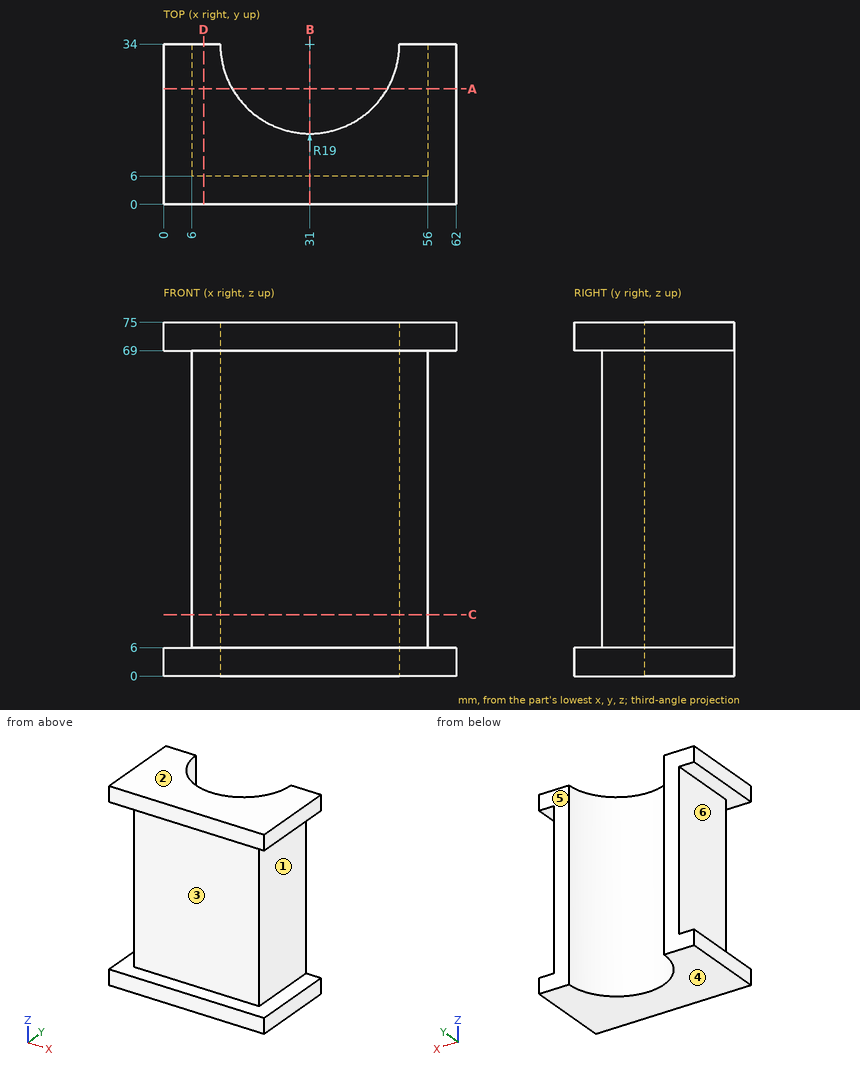
Design review of the part shown in the three views and the two pictorial views. Dimensions are in mm from the part's minimum x, y and z. A direction names the side the tool comes from. Round coordinates to 2 decimals unless told otherwise and drop trailing zeros. Order: outer loops, then holes, each group sorted by start corner. A loop starts at its lowest first (then second) coordinate and runs counter-clockwise, first axis right, second up. Notation, with made-up numbers: (47, 44.5) - (89, 44.5) arc R32 cw to (89, 79.5) - close; hole circle Ø4 at (54.25, 22.25). An arc over 180 degrees is marked (long way). Answer in a Markdown table with one row per item.
(1) Take a section at A-A on y = 24.5. Write out the cut boundary in (x, z), plus the area to 3 significant figures.
Result set:
| item | result |
|---|---|
| outline | (0, 0) - (14.55, 0) - (14.55, 75) - (0, 75) - (0, 69) - (6, 69) - (6, 6) - (0, 6) - close; (47.45, 0) - (62, 0) - (62, 6) - (56, 6) - (56, 69) - (62, 69) - (62, 75) - (47.45, 75) - close |
| area | 1,430 mm2 |
(2) For line 1 (Z direction, x = 44.5, y = 5.5); line 2 (X direction, y = 31.5, z = 12); line 3 (X direction, y = 9, z = 61.5), list the stretches that pass through material, from the lowest coordinate up. Write a range as from..to.
Result set:
| item | result |
|---|---|
| line 1 | z = 0..6, 69..75 |
| line 2 | x = 6..12.17, 49.83..56 |
| line 3 | x = 6..56 |
(3) Take a section at C-C on z = 13. Write out the cut boundary in (x, y), plus the area to 3 significant figures.
Result set:
| item | result |
|---|---|
| outline | (6, 6) - (56, 6) - (56, 34) - (50, 34) arc R19 cw to (12, 34) - (6, 34) - close |
| area | 833 mm2 |
(4) Mouldability with a two-part tool opening along Z and no side actions: class the marked faces 4, 5 and 6 as released by +Z, released by -Z, zero draft, split by the parting line, or undercut.
Result set:
| item | result |
|---|---|
| face 4 | released by -Z |
| face 5 | zero draft |
| face 6 | undercut |
(5) Clearance check with flat-ended pins moving along their axes: P1, Ø8.5, axis at y = 22, z = 26, coming from the +X side; P2, Ø2, axis at y = 16.5, z = 8, coming from the -X side; P3, Ø6, axis at x = 17.5, z = 8.5, coming from the +Y side. State where each tip first meets the part, or that it passes through.
Result set:
| item | result |
|---|---|
| P1 | stops at x = 56 |
| P2 | stops at x = 6 |
| P3 | stops at y = 24.58 |
(6) Take a section at B-B on x = 31. Write out the cut boundary in (y, z), plus the area to 3 significant figures.
Result set:
| item | result |
|---|---|
| outline | (0, 0) - (15, 0) - (15, 75) - (0, 75) - (0, 69) - (6, 69) - (6, 6) - (0, 6) - close |
| area | 747 mm2 |
(7) Take a section at D-D on x = 8.5. Write out the cut boundary in (y, z).
Result set:
| item | result |
|---|---|
| outline | (0, 0) - (34, 0) - (34, 75) - (0, 75) - (0, 69) - (6, 69) - (6, 6) - (0, 6) - close |
(8) Machinability: for the marked faces 1, 2 and 3, which of the approach directions +Z, -Z, +X, -X, +Y, -Y give a long, thin tool a straight path to every point of the face, cutting with its end or side? Answer none if there is none.
Result set:
| item | result |
|---|---|
| face 1 | +X, +Y, -Y |
| face 2 | +Z, +X, -X, +Y, -Y |
| face 3 | +X, -X, -Y |
